```python
from build123d import *

# Parameters (mm, degrees)
F0_W     = 30
F0_H     = 22
F1_DEPTH = 16
F2_W     = 38
F2_H     = 29
F2_W_2   = 30
F2_H_2   = 22
F3_DEPTH = 6
F4_R     = 1
F5_W     = 30
F5_H     = 10
F6_DEPTH = 12.5
F7_R     = 3


with BuildPart() as f1:
    # F0 (on Top) → F1 (new body)
    with BuildSketch(Plane.XY):
        Rectangle(F0_W, F0_H)
    extrude(amount=F1_DEPTH)

    # F2 (on face) → F3 (join)
    with BuildSketch(Plane.XY.offset(16)):
        Rectangle(F2_W, F2_H)
        Rectangle(F2_W_2, F2_H_2, mode=Mode.SUBTRACT)
        Rectangle(F2_W_2, F2_H_2)
    extrude(amount=F3_DEPTH)

    # F4
    f4_edges = [f1.edges().sort_by_distance(p)[0] for p in [
        (19, 0, 22),
        (0, 14.5, 22),
        (-19, 0, 22),
        (0, -14.5, 22),
    ]]
    fillet(f4_edges, radius=F4_R)

    # F5 (on Front) → F6 (join, symmetric)
    with BuildSketch(Plane.XZ):
        with Locations((0, 27)):
            Rectangle(F5_W, F5_H)
    extrude(amount=F6_DEPTH, both=True)

    # F7
    f7_edges = [f1.edges().sort_by_distance(p)[0] for p in [
        (0, 12.5, 32),
        (-15, 0, 32),
        (0, -12.5, 32),
        (15, 0, 32),
    ]]
    fillet(f7_edges, radius=F7_R)


solid = f1.part
```
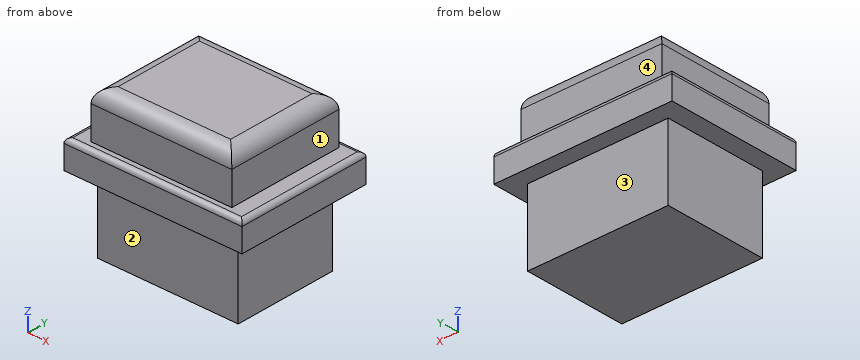
Geometry: final body of the model. Coordinates: model frame, mm. Face numbers are marked on the shaded views. A direction names the side the tool comes from. Round coordinates to 2 decimals unless told otherwise and drop trailing zeros. Loops run counter-clockwise (first coordinate to the right, second up) from the corner with the lowest first, then second, coordinate; pieces in that order, holes last. Notation, with made-up numbers: (24.25, 58.5) -> (41.25, 58.5) arc R10 cw to (41.25, 66.5) -> close; hole circle Ø8 at (65, -6). An arc over 180 degrees is marked (long way). Write each question's results on one line, items separated by ' | '.
Item 1: Cut plane D-D on x = 15.5. Return the cut outline in (y, z).
Answers below:
outline: (-14.5, 16) -> (14.5, 16) -> (14.5, 21) arc R1 ccw to (13.5, 22) -> (-13.5, 22) arc R1 ccw to (-14.5, 21) -> close
Item 2: Set-up query: the marked faces 1, 2, 3 and 4. Return all of +Z, -Z, +X, -X, +Y, -Y with unobstructed straight access to the full face (end or side cutting, diameter ignored); none if empty.
Answers below:
face 1: +Z, +X, +Y, -Y | face 2: -Z, +X, -X, -Y | face 3: -Z, +X, -X, +Y | face 4: +Z, +X, -X, +Y
Item 3: Cut plane B-B on x = -5.5. Return the cut outline in (y, z), and give its area (3 significant figures).
Answers below:
outline: (-14.5, 16) -> (-11, 16) -> (-11, 0) -> (11, 0) -> (11, 16) -> (14.5, 16) -> (14.5, 21) arc R1 ccw to (13.5, 22) -> (12.5, 22) -> (12.5, 29) arc R3 ccw to (9.5, 32) -> (-9.5, 32) arc R3 ccw to (-12.5, 29) -> (-12.5, 22) -> (-13.5, 22) arc R1 ccw to (-14.5, 21) -> close | area: 772 mm²
Item 4: Pin query (flat end, axial travel): pin 1 Ø5.5 at (y, z) = (1.5, 24) entering from -X; pin 2 Ø5 at (y, z) = (-7.5, 3.5) entering from +X; pin 3 Ø2 at (y, z) = (1, 13) entering from -X. Return the tip coordinate at first contact, or that it passes through.
Answers below:
pin 1: stops at x = -18.97 | pin 2: stops at x = 15 | pin 3: stops at x = -15
Item 5: Cut plane A-A on y = -8.25. Return the cut outline in (x, z), and give its area (3 significant figures).
Answers below:
outline: (-19, 16) -> (-15, 16) -> (-15, 0) -> (15, 0) -> (15, 16) -> (19, 16) -> (19, 21) arc R1 ccw to (18, 22) -> (15, 22) -> (15, 29) arc R3 ccw to (12, 32) -> (-12, 32) arc R3 ccw to (-15, 29) -> (-15, 22) -> (-18, 22) arc R1 ccw to (-19, 21) -> close | area: 1,000 mm²
Item 6: Cut plane C-C on z = 11.5. Return the cut outline in (x, y).
Answers below:
outline: (-15, -11) -> (15, -11) -> (15, 11) -> (-15, 11) -> close
Item 7: Line query: probe 1 along Y at (x, z) = (7, 24.5); probe 2 along X at (y, z) = (6.5, 10.5); probe 3 along Y at (x, z) = (-13, 2.5). Output: solid intervals per line, ascending. Write a range as [from, to].
Answers below:
probe 1: y = [-12.5, 12.5] | probe 2: x = [-15, 15] | probe 3: y = [-11, 11]
